```python
from build123d import *

# Parameters (mm, degrees)
F0_W     = 254
F0_H     = 127
F0_R     = 12.7
F1_DEPTH = 25.4
F3_DEPTH = 25.4


with BuildPart() as f1:
    # F0 (on Front) → F1 (new body)
    with BuildSketch(Plane.XZ):
        with Locations((-127, -63.5)):
            Rectangle(F0_W, F0_H)
        with Locations((-228.6, -101.6)):
            Circle(F0_R, mode=Mode.SUBTRACT)
        with Locations((-177.8, -101.6)):
            Circle(F0_R, mode=Mode.SUBTRACT)
        with Locations((-127, -101.6)):
            Circle(F0_R, mode=Mode.SUBTRACT)
        with Locations((-76.2, -101.6)):
            Circle(F0_R, mode=Mode.SUBTRACT)
        with Locations((-25.4, -101.6)):
            Circle(F0_R, mode=Mode.SUBTRACT)
        with Locations((-228.6, -63.5)):
            Circle(F0_R, mode=Mode.SUBTRACT)
        with Locations((-177.8, -63.5)):
            Circle(F0_R, mode=Mode.SUBTRACT)
        with Locations((-228.6, -25.4)):
            Circle(F0_R, mode=Mode.SUBTRACT)
        with Locations((-177.8, -25.4)):
            Circle(F0_R, mode=Mode.SUBTRACT)
        with Locations((-127, -63.5)):
            Circle(F0_R, mode=Mode.SUBTRACT)
        with Locations((-76.2, -63.5)):
            Circle(F0_R, mode=Mode.SUBTRACT)
        with Locations((-25.4, -63.5)):
            Circle(F0_R, mode=Mode.SUBTRACT)
        with Locations((-127, -25.4)):
            Circle(F0_R, mode=Mode.SUBTRACT)
        with Locations((-76.2, -25.4)):
            Circle(F0_R, mode=Mode.SUBTRACT)
        with Locations((-25.4, -25.4)):
            Circle(F0_R, mode=Mode.SUBTRACT)
    extrude(amount=F1_DEPTH)

    # F2 (on Right) → F3 (join)
    with BuildSketch(Plane.YZ):
        with BuildLine():
            ThreePointArc((3.218499, 49.117664), (11.833529, 24.029421), (-14.357061, 28.235564))
            ThreePointArc((-14.357061, 28.235564), (-15.469696, -7.155973), (8.052648, -33.622899))
            ThreePointArc((8.052648, -33.622899), (25.472188, -13.617942), (34.924857, -38.40273))
            ThreePointArc((34.924857, -38.40273), (66.131145, -21.670532), (77.291002, 11.933878))
            ThreePointArc((77.291002, 11.933878), (51.256432, 17.017165), (67.994353, 37.59581))
            ThreePointArc((67.994353, 37.59581), (37.900701, 56.255149), (3.218499, 49.117664))
        make_face()
    extrude(amount=F3_DEPTH)


solid = f1.part
```
Work out the finished part from the listing and answer in its coordinate system (mm). A direction names the side the tool comes from. Round coordinates to 2 decimals unless told otherwise and drop trailing zeros. Write each loop counter-clockwise with the first axis right and the second up, starting at its lowest first coordinate (ties: lowest second). Pieces come first, ordered by that corner, then holes. Notation, with made-up numbers: (83, 87.25) -> (127, 87.25) arc R12 cw to (127, 98.25) -> close; hole circle Ø3 at (-24.75, 10.5). An arc over 180 degrees is marked (long way). Write each question's results on one line, items separated by ' | '.
1) For a pull along Y with two mould halves and no side action, classify faces 3 (the cylindrical face through (12.522, 25.032, -13.546)), 4 (the flat face through (-129, -25.4, -77)), 5 (the cylindrical face through (-13.286, -12.522, -59.685)) as +Y half, -Y half, draft (parallel to the pull), parting line (faces both ways), or undercut.
Findings:
face 3: undercut | face 4: -Y half | face 5: draft
2) The part is cut by section B-B (z = -101.6). Write down the section's boundary in (x, y), and give its area (3 significant figures).
Findings:
outline: (-254, -25.4) -> (-241.3, -25.4) -> (-241.3, 0) -> (-254, 0) -> close; (-215.9, -25.4) -> (-190.5, -25.4) -> (-190.5, 0) -> (-215.9, 0) -> close; (-165.1, -25.4) -> (-139.7, -25.4) -> (-139.7, 0) -> (-165.1, 0) -> close; (-114.3, -25.4) -> (-88.9, -25.4) -> (-88.9, 0) -> (-114.3, 0) -> close; (-63.5, -25.4) -> (-38.1, -25.4) -> (-38.1, 0) -> (-63.5, 0) -> close; (-12.7, -25.4) -> (0, -25.4) -> (0, 0) -> (-12.7, 0) -> close | area: 3,230 mm²
3) Flat-ended cylindrical pins translate along their axes: pin 1 (6 mm diameter, centred on y = 46.5, z = 26, fed in from -X); pin 2 (3 mm diameter, centred on y = -14.5, z = -98, fed in from +X). Find the tip coordinate at first contact, or state that the pin passes through.
Findings:
pin 1: stops at x = 0 | pin 2: stops at x = 0
4) The part is cut by section D-D (y = 58). Write down the section's boundary in (x, z).
Findings:
outline: (0, -29.31) -> (25.4, -29.31) -> (25.4, 8.93) -> (0, 8.93) -> close; (0, 35.64) -> (25.4, 35.64) -> (25.4, 47.6) -> (0, 47.6) -> close
5) Which of the six approach directions +Z, -Z, +X, -X, +Y, -Y give full straight-line access (tool end or side, diameter ignored) to faces 1 (the cylindrical face through (-64.086, -12.522, -59.685)), 2 (the flat face through (0, -13, -64))?
Findings:
face 1: +Y, -Y | face 2: -Z, +X, -Y
6) Consider line 1 along Z through (x, y) = (-127, -16); line 2 along X through (y, z) = (-5, -101); line 3 along Z through (x, y) = (-57, -19). Determine where each line is inside the solid, lowest interval first. Write a range as [from, to].
Findings:
line 1: z = [-127, -114.3], [-88.9, -76.2], [-50.8, -38.1], [-12.7, 0] | line 2: x = [-254, -241.29], [-215.91, -190.49], [-165.11, -139.69], [-114.31, -88.89], [-63.51, -38.09], [-12.71, 0] | line 3: z = [-127, 0]
7) The part is cut by section C-C (z = -25.4). State how many separate pieces and enclosed holes the cut face has, and give its area (3 significant figures).
Findings:
separate pieces: 7 | enclosed holes: 0 | area: 4,140 mm²
8) The part is cut by section A-A (x = -21). Write down the section's boundary in (y, z).
Findings:
outline: (-25.4, -127) -> (0, -127) -> (0, -113.51) -> (-25.4, -113.51) -> close; (-25.4, -89.69) -> (0, -89.69) -> (0, -75.41) -> (-25.4, -75.41) -> close; (-25.4, -51.59) -> (0, -51.59) -> (0, -37.31) -> (-25.4, -37.31) -> close; (-25.4, -13.49) -> (0, -13.49) -> (0, 0) -> (-25.4, 0) -> close
